Geometry check sheet. Reference: the model listing, model coordinates, mm. Coordinates: 2 decimals unless noted, no trailing zeros. Write each loop counter-clockwise with the first axis right and the second up, starting at its lowest first coordinate (ties: lowest second). Pieces come first, ordered by that corner, then holes. Notation, with made-up numbers: (88, -14.75) -> (107, -14.75) arc R12 cw to (107, -8.75) -> close; hole circle Ø8 at (-27, 87.5). An arc over 180 degrees is marked (long way). Answer in a Markdown table with one row per item. Add a question column.
1. Cross-section at A-A on y = 0.95. Record the cut outline in (x, z).
2. Scan lines: L1, parallel to X at y = 1.8, z = 0; L2, parallel to X at y = 0.4, z = 60; L3, parallel to Z at x = 85, y = 1.9. Record each from-to range of solid material in increasing order. Write a range as from..to.
3. Cross-section at B-B on x = -27. Record the cut outline in (y, z).
4. Depth check by flat-ended pin: P1, Ø2.5, axis at x = -85, z = 0, coming from the +Y side; P2, Ø1.5, axis at x = -50.5, y = 2, coming from the +Z side; P3, Ø3, axis at x = 6.5, z = -50, coming from the -Y side. Enter the tip coordinate at first touch or a pass-through.
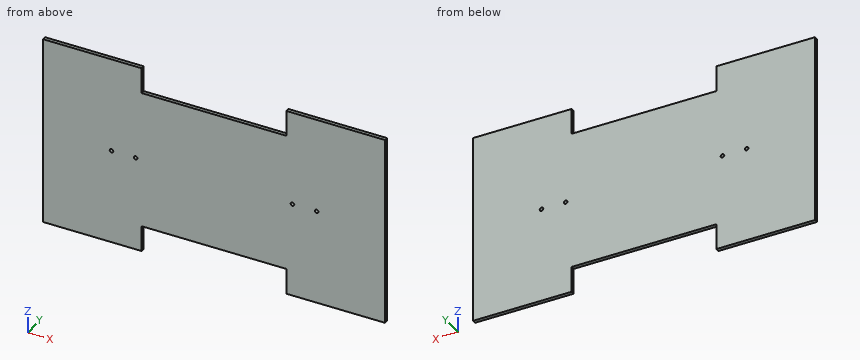
```python
from build123d import *

# Parameters (mm, degrees)
SKETCH1_W               = 283.5
SKETCH1_H               = 162
BOSS_EXTRUDE1_DEPTH     = 3
SKETCH2_W               = 120
SKETCH2_H               = 22
CUT_EXTRUDE1_DEPTH      = 3
CUT_EXTRUDE3_DEPTH      = 164.288280351
CUT_EXTRUDE3_DEPTH_BACK = 164.288280351
SKETCH4_R               = 1.5


with BuildPart() as part:
    # Sketch1 → Boss-Extrude1 (new body)
    with BuildSketch(Plane(origin=(0, 0, 0), x_dir=(1, 0, 0), z_dir=(0, 1, 0))):
        Rectangle(SKETCH1_W, SKETCH1_H)
    extrude(amount=BOSS_EXTRUDE1_DEPTH)

    # Sketch2 → Cut-Extrude1 (cut)
    with BuildSketch(Plane(origin=(0, 3, 0), x_dir=(1, 0, 0), z_dir=(0, 1, 0))):
        with Locations((0, -70)):
            Rectangle(SKETCH2_W, SKETCH2_H)
        with Locations((0, 70)):
            Rectangle(SKETCH2_W, SKETCH2_H)
    extrude(amount=-CUT_EXTRUDE1_DEPTH, mode=Mode.SUBTRACT)

    # Sketch4 → Cut-Extrude3 (cut, two sides: drawn at the far end of the back side and taken through both)
    with BuildSketch(Plane(origin=(0, 3, 0), x_dir=(1, 0, 0), z_dir=(0, 1, 0)).offset(-CUT_EXTRUDE3_DEPTH_BACK)):
        with Locations(Location((-85, 0, 0), (0, 0, 270))):
            Circle(SKETCH4_R)
        with Locations(Location((-65, 0, 0), (0, 0, 270))):
            Circle(SKETCH4_R)
        with Locations(Location((65, 0, 0), (0, 0, 270))):
            Circle(SKETCH4_R)
        with Locations(Location((85, 0, 0), (0, 0, 270))):
            Circle(SKETCH4_R)
    extrude(amount=CUT_EXTRUDE3_DEPTH + CUT_EXTRUDE3_DEPTH_BACK, mode=Mode.SUBTRACT)


solid = part.part
```
Results found:
| question | item | result |
|---|---|---|
| 1 | outline | (-141.75, -81) -> (-60, -81) -> (-60, -59) -> (60, -59) -> (60, -81) -> (141.75, -81) -> (141.75, 81) -> (60, 81) -> (60, 59) -> (-60, 59) -> (-60, 81) -> (-141.75, 81) -> close; hole circle Ø3 at (-85, 0); hole circle Ø3 at (-65, 0); hole circle Ø3 at (65, 0); hole circle Ø3 at (85, 0) |
| 2 | L1 | x = -141.75..-86.5, -83.5..-66.5, -63.5..63.5, 66.5..83.5, 86.5..141.75 |
| 2 | L2 | x = -141.75..-60, 60..141.75 |
| 2 | L3 | z = -81..-1.5, 1.5..81 |
| 3 | outline | (0, -59) -> (3, -59) -> (3, 59) -> (0, 59) -> close |
| 4 | P1 | passes through |
| 4 | P2 | stops at z = 59 |
| 4 | P3 | stops at y = 0 |
